Autodesk Fusion 360 part; units mm, degrees
sketch "Sketch1" plane through (0, 0, 0) normal (0, 0, 1) x (1, 0, 0)
  circle A0 centre (0, 0) radius 1.75
  circle A1 centre (10, 0) radius 1.775
  circle A2 centre (20, 0) radius 1.8
  circle A3 centre (30, 0) radius 1.825
  circle A4 centre (40, 0) radius 1.85
  line L0 (0, 0) -> (10, 0) construction
  line L1 (10, 0) -> (20, 0) construction
  line L2 (20, 0) -> (30, 0) construction
  line L3 (30, 0) -> (40, 0) construction
  circle A5 centre (50, 0) radius 1.875
  circle A6 centre (60, 0) radius 1.9
  circle A7 centre (70, 0) radius 1.925
  line L4 (40, 0) -> (50, 0) construction
  line L5 (50, 0) -> (60, 0) construction
  line L6 (60, 0) -> (70, 0) construction
  line L7 (-50, 0) -> (-40, 0) construction
  line L8 (-40, 0) -> (-30, 0) construction
  circle A8 centre (-40, 0) radius 1.65
  line L9 (-10, 0) -> (0, 0) construction
  circle A9 centre (-50, 0) radius 1.625
  circle A10 centre (-30, 0) radius 1.675
  circle A11 centre (-60, 0) radius 1.6
  circle A12 centre (-20, 0) radius 1.7
  line L10 (-30, 0) -> (-20, 0) construction
  line L11 (-60, 0) -> (-50, 0) construction
  line L12 (-20, 0) -> (-10, 0) construction
  circle A13 centre (-10, 0) radius 1.725
  line L13 (0, 0) -> (0, 10) construction
  circle A14 centre (-40, 10) radius 0.95
  line L14 (-50, 10) -> (-40, 10) construction
  line L15 (20, 10) -> (30, 10) construction
  circle A15 centre (20, 10) radius 1.1
  line L16 (-30, 10) -> (-20, 10) construction
  circle A16 centre (0, 10) radius 1.05
  circle A17 centre (-50, 10) radius 0.925
  line L17 (-60, 10) -> (-50, 10) construction
  line L18 (40, 10) -> (50, 10) construction
  line L19 (-40, 10) -> (-30, 10) construction
  circle A18 centre (10, 10) radius 1.075
  circle A19 centre (-30, 10) radius 0.975
  line L20 (-20, 10) -> (-10, 10) construction
  circle A20 centre (60, 10) radius 1.2
  circle A21 centre (70, 10) radius 1.225
  line L21 (60, 10) -> (70, 10) construction
  circle A22 centre (30, 10) radius 1.125
  line L22 (50, 10) -> (60, 10) construction
  circle A23 centre (40, 10) radius 1.15
  circle A24 centre (50, 10) radius 1.175
  line L23 (30, 10) -> (40, 10) construction
  circle A25 centre (-10, 10) radius 1.025
  line L24 (-10, 10) -> (0, 10) construction
  line L25 (0, 10) -> (10, 10) construction
  circle A26 centre (-20, 10) radius 1
  circle A27 centre (-60, 10) radius 0.9
  line L26 (10, 10) -> (20, 10) construction
  line L27 (0, 0) -> (0, -10) construction
  line L28 (0, -10) -> (10, -10) construction
  circle A28 centre (30, -10) radius 1.575
  circle A29 centre (20, -10) radius 1.55
  circle A30 centre (40, -10) radius 1.6
  line L29 (50, -10) -> (60, -10) construction
  circle A31 centre (70, -10) radius 1.675
  circle A32 centre (10, -10) radius 1.525
  line L30 (20, -10) -> (30, -10) construction
  circle A33 centre (0, -10) radius 1.5
  line L31 (-20, -10) -> (-10, -10) construction
  circle A34 centre (-10, -10) radius 1.475
  circle A35 centre (-20, -10) radius 1.45
  line L32 (-10, -10) -> (0, -10) construction
  circle A36 centre (-40, -10) radius 1.4
  circle A37 centre (-60, -10) radius 1.35
  line L33 (-60, -10) -> (-50, -10) construction
  line L34 (-30, -10) -> (-20, -10) construction
  circle A38 centre (-50, -10) radius 1.375
  line L35 (-40, -10) -> (-30, -10) construction
  line L36 (-50, -10) -> (-40, -10) construction
  circle A39 centre (-30, -10) radius 1.425
  circle A40 centre (50, -10) radius 1.625
  line L37 (10, -10) -> (20, -10) construction
  line L38 (40, -10) -> (50, -10) construction
  line L39 (60, -10) -> (70, -10) construction
  line L40 (30, -10) -> (40, -10) construction
  circle A41 centre (60, -10) radius 1.65
  line L41 (73.5, 3.833) -> (-63.5, 3.833)
  line L42 (-63.5, 3.833) -> (-63.5, -13.5)
  line L43 (-63.5, -13.5) -> (73.5, -13.5)
  line L44 (73.5, -13.5) -> (73.5, 3.833)
  point P0 (-60, 0)
  point P1 (-60, 10)
  point P2 (0, 10)
  point P3 (0, 10)
  point P4 (0, -10)
  point P5 (-60, -10)
  point P6 (0, -10)
  point P7 (0, -10)
  point P8 (5, 0)
  dimension "d1" = 3.5
  dimension "d2" = 10
  dimension "d3" = 3.55
  dimension "d4" = 3.6
  dimension "d5" = 3.65
  dimension "d6" = 3.7
  dimension "d7" = 3.75
  dimension "d8" = 3.8
  dimension "d9" = 3.85
  dimension "d10" = 3.2
  dimension "d11" = 10
  dimension "d12" = 3.25
  dimension "d13" = 3.3
  dimension "d14" = 3.35
  dimension "d15" = 3.4
  dimension "d16" = 3.45
  dimension "d18" = 10
  dimension "d19" = 2.1
  dimension "d20" = 10
  dimension "d21" = 2.15
  dimension "d22" = 2.2
  dimension "d23" = 2.25
  dimension "d24" = 2.3
  dimension "d25" = 2.35
  dimension "d26" = 2.4
  dimension "d27" = 2.45
  dimension "d28" = 1.8
  dimension "d29" = 10
  dimension "d30" = 1.85
  dimension "d31" = 1.9
  dimension "d32" = 1.95
  dimension "d33" = 2
  dimension "d34" = 2.05
  dimension "d35" = 3
  dimension "d36" = 10
  dimension "d37" = 3.05
  dimension "d38" = 3.1
  dimension "d39" = 3.15
  dimension "d40" = 3.2
  dimension "d41" = 3.25
  dimension "d42" = 3.3
  dimension "d43" = 3.35
  dimension "d44" = 2.7
  dimension "d45" = 10
  dimension "d46" = 2.75
  dimension "d47" = 2.8
  dimension "d48" = 2.85
  dimension "d49" = 2.9
  dimension "d50" = 2.95
  dimension "d51" = 137
extrude "Extrude1" add sketch "Sketch1" along normal blind 10 contours L41 L42 L43 L44
fillet "Fillet1" radius 3 4 edges at (73.5, -13.5, 5) (73.5, 3.833, 5) (-63.5, -13.5, 5) (-63.5, 3.833, 5)
equation "d2 = d18"
equation "d3 = d1 + 0.05 mm"
equation "d4 = d3 + 0.05 mm"
equation "d5 = d4 + 0.05 mm"
equation "d6 = d5 + 0.05 mm"
equation "d7 = d6 + 0.05 mm"
equation "d8 = d7 + 0.05 mm"
equation "d9 = d8 + 0.05 mm"
equation "d10 = d12 - 0.05 mm"
equation "d11 = d2"
equation "d12 = d13 - 0.05 mm"
equation "d13 = d14 - 0.05 mm"
equation "d14 = d15 - 0.05 mm"
equation "d15 = d16 - 0.05 mm"
equation "d16 = d1 - 0.05 mm"
equation "d20 = d2"
equation "d21 = d19 + 0.05 mm"
equation "d22 = d19 + 0.1 mm"
equation "d23 = d19 + 0.15 mm"
equation "d24 = d19 + 0.2 mm"
equation "d25 = d19 + 0.25 mm"
equation "d26 = d19 + 0.3 mm"
equation "d27 = d19 + 0.35 mm"
equation "d28 = d19 - 0.3 mm"
equation "d29 = d2"
equation "d30 = d19 - 0.25 mm"
equation "d31 = d19 - 0.2 mm"
equation "d32 = d19 - 0.15 mm"
equation "d33 = d19 - 0.1 mm"
equation "d34 = d19 - 0.05 mm"
equation "d36 = d2"
equation "d37 = d35 + 0.05 mm"
equation "d38 = d37 + 0.05 mm"
equation "d39 = d38 + 0.05 mm"
equation "d40 = d39 + 0.05 mm"
equation "d41 = d40 + 0.05 mm"
equation "d42 = d41 + 0.05 mm"
equation "d43 = d42 + 0.05 mm"
equation "d44 = d46 - 0.05 mm"
equation "d45 = d2"
equation "d46 = d47 - 0.05 mm"
equation "d47 = d48 - 0.05 mm"
equation "d48 = d49 - 0.05 mm"
equation "d49 = d50 - 0.05 mm"
equation "d50 = d35 - 0.05 mm"
Check sheet for the modelled part. Datum: model origin and axes. Units: mm. Coordinates: 2 decimals unless noted, no trailing zeros. Write each loop counter-clockwise with the first axis right and the second up, starting at its lowest first coordinate (ties: lowest second). Pieces come first, ordered by that corner, then holes. Notation, with made-up numbers: M -3,28.5 L 39,28.5 A26 ccw 39,52.5 Z; hole C -11,63.5 d10. An arc over 180 degrees is marked long. Answer as CSV lines item,"result".
Q1. Mould release check, pull along Y, two halves, no side actions. Record for faces 1 (the face through (11.455, -10.458, 4.93)), 2 (the face through (4, -13.5, 5)), 3 (the face through (-62.598, 2.978, 5.07)): released by +Y, released by -Y, zero draft, split by the parting line, or undercut.
Check result:
face 1,"undercut"
face 2,"released by -Y"
face 3,"released by +Y"
Q2. Cross-section at C-C (z = 6). Count the separate pieces of the cut face and the enclosed holes in it, then the cut area to 3 significant figures.
Check result:
separate pieces,"1"
enclosed holes,"28"
area,"2,130 mm^2"
Q3. Cross-section at A-A (x = -10). Record the boundary of the cut face in (y, z) (3 decimals).
Check result:
outline,"M -13.5,0 L -11.475,0 L -11.475,10 L -13.5,10 Z; M -8.525,0 L -1.725,0 L -1.725,10 L -8.525,10 Z; M 1.725,0 L 3.833,0 L 3.833,10 L 1.725,10 Z"
Q4. Material ranges on probe 1 along Y at (x, z) = (0, 6.5); probe 2 along Y at (x, z) = (40, 6.5); probe 3 along X at (y, z) = (-12, 6.75), recorded low to high. Write a range as from..to.
Check result:
probe 1,"-13.5..-11.5, -8.5..-1.75, 1.75..3.83"
probe 2,"-13.5..-11.6, -8.4..-1.85, 1.85..3.83"
probe 3,"-63.1..73.1"
Q5. Cross-section at B-B (x = 60). Record the boundary of the cut face in (y, z), then the cut area to 3 significant figures.
Check result:
outline,"M -13.5,0 L -11.65,0 L -11.65,10 L -13.5,10 Z; M -8.35,0 L -1.9,0 L -1.9,10 L -8.35,10 Z; M 1.9,0 L 3.83,0 L 3.83,10 L 1.9,10 Z"
area,"102 mm^2"
Q6. Go/stop test with a flat-tipped pin: pin 1 (2.5 mm diameter, centred on x = -60, y = -10, fed in from -Z). Record where the tip stops, or that it passes through.
Check result:
pin 1,"through"
